The model under review builds one solid part; all positions refer to its coordinate system, in mm. Face numbers are marked on the shaded views. A direction names the side the tool comes from. Coordinates: 2 decimals unless noted, no trailing zeros. Order: outer loops, then holes, each group sorted by start corner. A loop starts at its lowest first (then second) coordinate and runs counter-clockwise, first axis right, second up.
```python
from build123d import *

# Parameters (mm, degrees)
F1_DEPTH = 60
F2_DEPTH = 3


with BuildPart() as f1:
    # F0 (on Top) → F1 (new body)
    with BuildSketch(Plane.XY):
        Polygon((27.5, -47.631397), (55, 0), (27.5, 47.631397), (-27.5, 47.631397), (-55, 0), (-27.5, -47.631397), align=None)
        Polygon((26, 45.033321), (52, 0), (26, -45.033321), (-26, -45.033321), (-52, 0), (-26, 45.033321), align=None, mode=Mode.SUBTRACT)
    extrude(amount=F1_DEPTH)

    # F0 (on Top) → F2 (join)
    with BuildSketch(Plane.XY):
        Polygon((26, -45.033321), (52, 0), (26, 45.033321), (-26, 45.033321), (-52, 0), (-26, -45.033321), align=None)
    extrude(amount=F2_DEPTH)


solid = f1.part
```
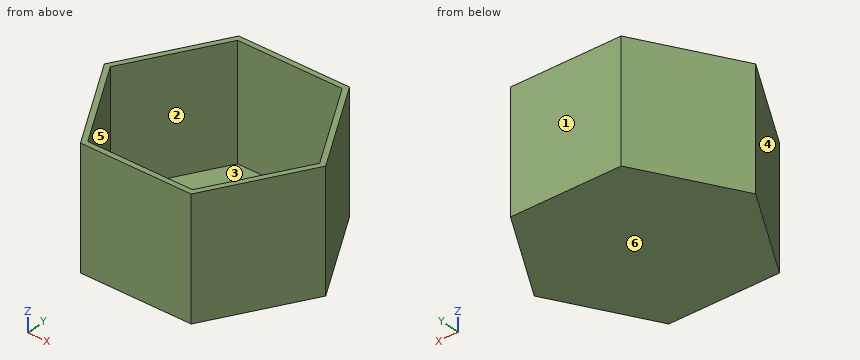
(1) Wall thickness on probe 1 along Y at (x, z) = (-6.5, 33.5); probe 2 along Z at (x, y) = (-4.5, -28); probe 3 along X at (y, z) = (37, 41.5): over which ranges is each line inside the solid? List them lowest first.
A:
probe 1: y = -47.63 to -45.03, 45.03 to 47.63
probe 2: z = 0 to 3
probe 3: x = -33.64 to -30.64, 30.64 to 33.64
(2) For pin 1 Ø3 at (y, z) = (-15, 10) entering from +X; pin 2 Ø2 at (x, y) = (-43.5, -1) entering from +Z; pin 3 Ø4 at (x, z) = (31.5, 52) entering from -Y, all flat-tipped, find the tip position at first contact; note any pin that passes through.
A:
pin 1: stops at x = 47.21
pin 2: stops at z = 3
pin 3: stops at y = -44.17
(3) Draft analysis for pull direction Y (two halves, no side actions). For the marked faces 3, 4, 5 and 6, state which applies: released by +Y, released by -Y, zero draft, split by the parting line, or undercut.
A:
face 3: undercut
face 4: released by -Y
face 5: undercut
face 6: zero draft
(4) We need section A-A, the plane z = 50. Write out the cut boundary in (x, y), and give its area (3 significant figures).
A:
outline: (-55, 0) - (-27.5, -47.63) - (27.5, -47.63) - (55, 0) - (27.5, 47.63) - (-27.5, 47.63) - close; hole (-52, 0) - (-26, -45.03) - (26, -45.03) - (52, 0) - (26, 45.03) - (-26, 45.03) - close
area: 834 mm2
(5) We need section B-B, the plane x = 11. Write out the cut boundary in (y, z), and give its area (3 significant figures).
A:
outline: (-47.63, 0) - (47.63, 0) - (47.63, 60) - (45.03, 60) - (45.03, 3) - (-45.03, 3) - (-45.03, 60) - (-47.63, 60) - close
area: 582 mm2
(6) Machinability: for the marked faces 1 and 2, which of the approach directions +Z, -Z, +X, -X, +Y, -Y give a long, thin tool a straight path to every point of the face, cutting with its end or side? Answer none if there is none.
A:
face 1: +Z, -Z, +X, -X, +Y
face 2: +Z
(7) We need section C-C, the plane y = 21. Write out the cut boundary in (x, z), and give its area (3 significant figures).
A:
outline: (-42.88, 0) - (42.88, 0) - (42.88, 60) - (39.88, 60) - (39.88, 3) - (-39.88, 3) - (-39.88, 60) - (-42.88, 60) - close
area: 599 mm2
